```python
from build123d import *

# Parameters (mm, degrees)
SKETCH1_W               = 86.36
SKETCH1_H               = 6.35
BOSS_EXTRUDE1_DEPTH     = 25.4
BOSS_EXTRUDE2_DEPTH     = 25.4
SKETCH3_R               = 7.62
SKETCH3_R_2             = 1.651
CUT_EXTRUDE3_DEPTH      = 25.4
SKETCH4_R               = 20
CUT_EXTRUDE4_DEPTH      = 19.05
SKETCH6_W               = 40
SKETCH6_H               = 10.16
CUT_EXTRUDE6_DEPTH      = 19.05
BOSS_EXTRUDE3_START     = -25.4
SKETCH7_W               = 15.24
SKETCH7_H               = 16.19
SKETCH7_R               = 4
BOSS_EXTRUDE3_DEPTH     = 25.4
FILLET1_R               = 6.35
SKETCH9_R               = 1.5875
CUT_EXTRUDE7_DEPTH      = 62.801201445
CUT_EXTRUDE8_REACH      = 56.934
CUT_EXTRUDE8_END_RADIUS = 4
SKETCH11_R              = 1.5875


with BuildPart() as part:
    # Sketch1 → Boss-Extrude1 (new body)
    with BuildSketch(Plane.XY):
        Rectangle(SKETCH1_W, SKETCH1_H)
    extrude(amount=BOSS_EXTRUDE1_DEPTH)

    # Sketch2 → Boss-Extrude2 (add)
    with BuildSketch(Plane.XY.offset(25.4)):
        with BuildLine():
            ThreePointArc((20, 19.365), (0, 39.365), (-20, 19.365))
            ThreePointArc((-20, 19.365), (-17.816396252, 10.277864885), (-11.742397541, 3.175))
            Line((-11.742397541, 3.175), (11.742397541, 3.175))
            ThreePointArc((11.742397541, 3.175), (17.816396252, 10.277864885), (20, 19.365))
        make_face()
        with BuildLine():
            Line((11.742397541, 3.175), (-11.742397541, 3.175))
            ThreePointArc((-11.742397541, 3.175), (0, -0.635), (11.742397541, 3.175))
        make_face()
        with BuildLine():
            ThreePointArc((-11.742397541, 3.175), (-17.816396252, 10.277864885), (-20, 19.365))
            Line((-20, 19.365), (-20, 3.175))
            Line((-20, 3.175), (-11.742397541, 3.175))
        make_face()
        with BuildLine():
            Line((20, 3.175), (20, 19.365))
            ThreePointArc((20, 19.365), (17.816396252, 10.277864885), (11.742397541, 3.175))
            Line((11.742397541, 3.175), (20, 3.175))
        make_face()
    extrude(amount=-BOSS_EXTRUDE2_DEPTH)

    # Sketch3 → Cut-Extrude3 (cut)
    with BuildSketch(Plane.XY.offset(25.4)):
        with Locations((0, 12.253)):
            Circle(SKETCH3_R)
        with Locations((-7.79423, 32.755818299)):
            Circle(SKETCH3_R_2)
        with Locations((7.79423, 32.755818299)):
            Circle(SKETCH3_R_2)
        with Locations((-15.58846, 19.365)):
            Circle(SKETCH3_R_2)
        with Locations((15.58846, 19.365)):
            Circle(SKETCH3_R_2)
    extrude(amount=-CUT_EXTRUDE3_DEPTH, mode=Mode.SUBTRACT)

    # Sketch4 → Cut-Extrude4 (cut)
    with BuildSketch(Plane(origin=(0, 0, 0), x_dir=(-1, 0, 0), z_dir=(0, 0, -1))):
        with Locations((0, 19.365)):
            Circle(SKETCH4_R)
    extrude(amount=-CUT_EXTRUDE4_DEPTH, mode=Mode.SUBTRACT)

    # Sketch6 → Cut-Extrude6 (cut)
    with BuildSketch(Plane(origin=(0, 0, 0), x_dir=(-1, 0, 0), z_dir=(0, 0, -1))):
        with Locations((0, 14.285)):
            Rectangle(SKETCH6_W, SKETCH6_H)
    extrude(amount=-CUT_EXTRUDE6_DEPTH, mode=Mode.SUBTRACT)

    # Sketch7 → Boss-Extrude3 (add)
    with BuildSketch(Plane.XY.offset(25.4).offset(BOSS_EXTRUDE3_START)):
        with Locations((-27.62, 11.27)):
            Rectangle(SKETCH7_W, SKETCH7_H)
        with Locations((-26.9875, 11.999)):
            Circle(SKETCH7_R, mode=Mode.SUBTRACT)
    boss_extrude3 = extrude(amount=BOSS_EXTRUDE3_DEPTH)

    # Mirror2: Boss-Extrude3 across plane
    add(boss_extrude3.mirror(Plane(origin=(0, 0, 0), x_dir=(0, 0, 1), z_dir=(1, 0, 0))))

    # Fillet1
    fillet1_edges = [part.edges().sort_by_distance(p)[0] for p in [
        (-35.24, 19.365, 12.7),
        (35.24, 19.365, 12.7),
    ]]
    fillet(fillet1_edges, radius=FILLET1_R)

    # Sketch9 → Cut-Extrude7 (cut, through all)
    with BuildSketch(Plane(origin=(0, 3.175, 0), x_dir=(1, 0, 0), z_dir=(0, 1, 0))):
        with Locations(Location((-39.21, -6.35, 0), (0, 0, 180))):
            Circle(SKETCH9_R)
        with Locations(Location((-39.21, -19.05, 0), (0, 0, 180))):
            Circle(SKETCH9_R)
    cut_extrude7 = extrude(amount=-CUT_EXTRUDE7_DEPTH, mode=Mode.SUBTRACT)

    # Mirror3: Cut-Extrude7 across plane
    add(cut_extrude7.mirror(Plane(origin=(0, 0, 0), x_dir=(0, 0, 1), z_dir=(1, 0, 0))), mode=Mode.SUBTRACT)

    # Cut-Extrude8: up to this cylinder (the profile starts outside it)
    cut_extrude8_end = Plane(origin=(-26.9875, 11.999, 9.525), z_dir=(0, 0, 1)) * Cylinder(CUT_EXTRUDE8_END_RADIUS, 122.868, mode=Mode.PRIVATE)
    # Sketch11 → Cut-Extrude8 (cut, up to the surface)
    with BuildSketch(Plane(origin=(0, 19.365, 0), x_dir=(1, 0, 0), z_dir=(0, 1, 0)), mode=Mode.PRIVATE) as cut_extrude8_sk1:
        with Locations(Location((-27.62, -9.525, 0), (0, 0, 270))):
            Circle(SKETCH11_R)
    cut_extrude8_tool1 = extrude(cut_extrude8_sk1.sketch, amount=-CUT_EXTRUDE8_REACH, mode=Mode.PRIVATE) - cut_extrude8_end
    cut_extrude8 = cut_extrude8_tool1.solids().sort_by_distance((-27.62, 19.365, 9.525))[0]
    add(cut_extrude8, mode=Mode.SUBTRACT)

    # Mirror4: Cut-Extrude8 across plane
    add(cut_extrude8.mirror(Plane(origin=(0, 0, 0), x_dir=(0, 0, 1), z_dir=(1, 0, 0))), mode=Mode.SUBTRACT)


solid = part.part
```
Input: part model. Units: mm. Frame: model coordinates. A direction names the side the tool comes from. Coordinates: 2 decimals unless noted, no trailing zeros. Order: outer loops, then holes, each group sorted by start corner. A loop starts at its lowest first (then second) coordinate and runs counter-clockwise, first axis right, second up. Notation, with made-up numbers: (67.25, 37.5) - (120.25, 37.5) arc R19 ccw to (120.25, 57.5) - close; hole circle Ø10 at (73.25, 44). An arc over 180 degrees is marked (long way). Return JSON: item names as keys, results as strings.
Q1. Cut plane D-D (x = 24.5). Return loops of the section in (y, z) (3 decimals), then the cut area to 3 significant figures.
The answers:
{"outline": "(-3.175, 0) - (8.867, 0) - (8.867, 25.4) - (-3.175, 25.4) - close; (15.131, 0) - (19.365, 0) - (19.365, 25.4) - (15.131, 25.4) - close", "area": "413 mm2"}
Q2. Ray query, probe 1 along Z at (x, y) = (-27.62, 16.3); probe 2 along Z at (x, y) = (39.21, 0.25); probe 3 along X at (y, z) = (15.5, 13). Return the intervals inside material, ascending.
The answers:
{"probe 1": "z = 0 to 7.94, 11.11 to 25.4", "probe 2": "z = 0 to 4.76, 7.94 to 17.46, 20.64 to 25.4", "probe 3": "x = -34.73 to -28.92, -25.05 to -20, 20 to 25.05, 28.92 to 34.73"}
Q3. Cut plane C-C (z = 23.5). State how many separate pieces and enclosed holes the cut face has, then the cut area to 3 significant figures.
The answers:
{"separate pieces": "1", "enclosed holes": "7", "area": "1,980 mm2"}
Q4. Cut plane A-A (x = 0). Return loops of the section in (y, z) (3 decimals).
The answers:
{"outline": "(-3.175, 0) - (-0.635, 0) - (-0.635, 19.05) - (4.633, 19.05) - (4.633, 25.4) - (-3.175, 25.4) - close; (19.873, 19.05) - (39.365, 19.05) - (39.365, 25.4) - (19.873, 25.4) - close"}
Q5. First-contact query: pin 1 (8 mm diameter, centred on x = -14.5, y = 29.5, fed in from -Z); pin 2 (8.5 mm diameter, centred on x = 37.5, z = 16.5, fed in from +Y); pin 3 (2 mm diameter, centred on x = -26, z = 16, fed in from +Y) (3 decimals); pin 4 (6.5 mm diameter, centred on x = 26.99, y = 12, fed in from +Z). Flat tips, straight axial feed; report the tip coordinate or a pass-through.
The answers:
{"pin 1": "stops at z = 19.05", "pin 2": "stops at y = 17.63", "pin 3": "stops at y = 19.365", "pin 4": "passes through"}
Q6. Access query for faces 1 (the cylindrical face through (40.724, 0.044, 6.827)), 2 (the flat face through (-35.24, 8, 13)), 3 (the flat face through (39, 3.175, 13)), 4 (the flat face through (19, 9.205, 9)), 5 (the cylindrical face through (-29.17, 17.37, 9.18)). Directions: +Z, -Z, +X, -X, +Y, -Y. A direction counts if a zero-diameter tool reaches every point of the face in a straight line with its end or side. Return the directions, or none.
The answers:
{"face 1": "+Y, -Y", "face 2": "+Z, -Z, -X, +Y", "face 3": "+Z, -Z, +X, +Y", "face 4": "-Z, +Y", "face 5": "+Y"}
Q7. Draft query along X for faces 6 (the flat face through (-4, 20, 19.05)), 7 (the flat face through (43.18, 0, 13)), 8 (the flat face through (25, 19.365, 13)). Return one class per face: +X half, -X half, draft (parallel to the pull), parting line (faces both ways), or undercut.
The answers:
{"face 6": "undercut", "face 7": "+X half", "face 8": "draft"}
Q8. Cut plane B-B (x = -27.62). Return loops of the section in (y, z) (1 decimal).
The answers:
{"outline": "(-3.2, 0) - (8, 0) - (8, 25.4) - (-3.2, 25.4) - close; (15.9, 0) - (19.4, 0) - (19.4, 7.9) - (15.9, 7.9) - close; (15.9, 11.1) - (19.4, 11.1) - (19.4, 25.4) - (15.9, 25.4) - close"}
